Answer from the drawing. Dimensions are ordinates in mm from the lowest x, y and z of the part. A direction names the side the tool comes from. Give positions to 0.01 mm unless a question says otherwise; leave off trailing zeros. Write each loop counter-clockwise with the first axis right and the second up, starting at its lowest first coordinate (ties: lowest second). Pieces come first, ordered by that corner, then holes. Notation, with made-up numbers: (32.5, 23.5) - (49.5, 23.5) arc R15 ccw to (49.5, 31.5) - close; hole circle Ø1 at (85.25, 81.25). An arc over 180 degrees is marked (long way). Write item = value, one per line.
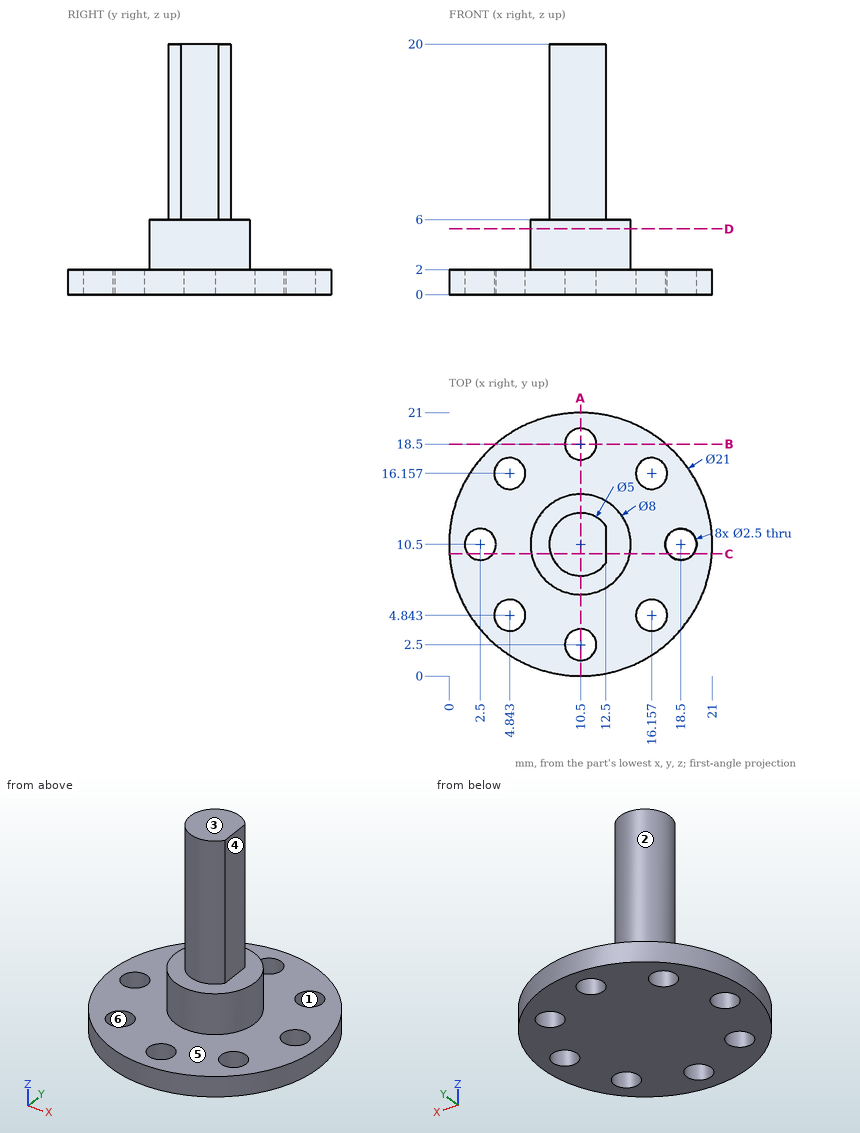
1. Find section C-C, the plane y = 9.75. Give the vertices of the cut face in (x, z) (3 decimals), then the cut area to 3 significant figures.
Solution:
outline = (0.027, 0) - (1.5, 0) - (1.5, 2) - (0.027, 2) - close; (3.5, 0) - (17.5, 0) - (17.5, 2) - (14.429, 2) - (14.429, 6) - (12.5, 6) - (12.5, 20) - (8.115, 20) - (8.115, 6) - (6.571, 6) - (6.571, 2) - (3.5, 2) - close; (19.5, 0) - (20.973, 0) - (20.973, 2) - (19.5, 2) - close
area = 127 mm^2
2. Find section B-B, the plane y = 18.5. Give the vertices of the cut face in (x, z), then the cut area to 3 significant figures.
Solution:
outline = (3.7, 0) - (9.25, 0) - (9.25, 2) - (3.7, 2) - close; (11.75, 0) - (17.3, 0) - (17.3, 2) - (11.75, 2) - close
area = 22.2 mm^2
3. For a pull along X with two mould halves and no side action, classify the marked faces 1, 2 and 3 as pulls with the +X half, pulls with the -X half, needs draft (parallel to the pull), parting line crosses it, or undercut.
Solution:
face_1 = undercut
face_2 = parting line crosses it
face_3 = needs draft
4. Find section A-A, the plane x = 10.5. Give the vertices of the cut face in (y, z).
Solution:
outline = (0, 0) - (1.25, 0) - (1.25, 2) - (0, 2) - close; (3.75, 0) - (17.25, 0) - (17.25, 2) - (14.5, 2) - (14.5, 6) - (13, 6) - (13, 20) - (8, 20) - (8, 6) - (6.5, 6) - (6.5, 2) - (3.75, 2) - close; (19.75, 0) - (21, 0) - (21, 2) - (19.75, 2) - close
5. Straight lines are drawn through the part: line 1 (Z direction, x = 6.5, y = 20); line 2 (Y direction, x = 2.5, z = 0.4); line 3 (Z direction, x = 8.75, y = 7.5). For each, find the intervals that lie inside material, in ascending order.
Solution:
line_1 = 0 to 2
line_2 = 3.7 to 9.25, 11.75 to 17.3
line_3 = 0 to 6
6. Given pin 1 (3 mm diameter, centred on x = 7, z = 12, fed in from -Y); pin 2 (1 mm diameter, centred on x = 11, z = 12.5, fed in from +Y); pin 3 (3 mm diameter, centred on x = 10.5, y = 2.5, fed in from +Z), each flat-ended and moving along its own axis, determine where each tip first touches the part or whether it passes through.
Solution:
pin_1 = 9
pin_2 = 13
pin_3 = 2
7. Find section D-D, the plane z = 5.25. Give the vertices of the cut face in (x, y).
Solution:
outline = circle Ø8 at (10.5, 10.5)
8. A tool of negligible diameter and unlimited length cuts with its end or side. For the marked faces 4, 5 and 6, from which of +Z, -Z, +X, -X, +Y, -Y can it reach the whole face along a straight path? Write none if from no direction.
Solution:
face_4 = +Z, +X, +Y, -Y
face_5 = +Z
face_6 = +Z, -Z
